The model under review builds one solid part; all positions refer to its coordinate system, in mm. Round coordinates to 2 decimals unless told otherwise and drop trailing zeros. Write each loop counter-clockwise with the first axis right and the second up, starting at its lowest first coordinate (ties: lowest second). Pieces come first, ordered by that corner, then holes. Notation, with made-up numbers: (52, 51) -> (65, 51) arc R15 ccw to (65, 76) -> close; hole circle Ø10 at (26, -19.5). An arc over 180 degrees is marked (long way). Answer in a Markdown table with one row per item. Add a question column.
```python
from build123d import *

# Parameters (mm, degrees)
SKETCH_1_W          = 213
SKETCH_1_H          = 200
EXTRUDE_1_DEPTH     = 5
SKETCH_2_R          = 2
SKETCH_2_R_2        = 6
CUT_EXTRUDE_1_DEPTH = 147.175408328
SKETCH_3_W          = 213
SKETCH_3_H          = 12.904797871
CUT_EXTRUDE_2_DEPTH = 147.175408328
SKETCH_4_W          = 28
SKETCH_4_H          = 35
CUT_EXTRUDE_3_DEPTH = 147.175408328
FILLET_1_R          = 5
SKETCH_5_W          = 42
SKETCH_5_H          = 70.904797871
EXTRUDE_2_DEPTH     = 5
FILLET_2_R          = 20
SKETCH_6_R          = 2
CUT_EXTRUDE_4_DEPTH = 202.434108173
SKETCH_7_R          = 2
CUT_EXTRUDE_5_DEPTH = 202.434108173
SKETCH_8_W          = 20
SKETCH_8_H          = 22
CUT_EXTRUDE_6_DEPTH = 202.434108173
FILLET_3_R          = 3
SKETCH_9_W          = 18
SKETCH_9_H          = 22
CUT_EXTRUDE_7_DEPTH = 202.434108173
SKETCH_10_R         = 1.5
CUT_EXTRUDE_8_DEPTH = 202.434108173
FILLET_4_R          = 10
SKETCH_11_W         = 115
SKETCH_11_H         = 73
CUT_EXTRUDE_9_DEPTH = 202.434108173
FILLET_5_R          = 5


with BuildPart() as part:
    # 草图1 → 凸台-拉伸1 (new body)
    with BuildSketch(Plane(origin=(0, 0, 0), x_dir=(1, 0, 0), z_dir=(0, 1, 0))):
        Rectangle(SKETCH_1_W, SKETCH_1_H)
    extrude(amount=EXTRUDE_1_DEPTH)

    # 草图2 → 切除-拉伸1 (cut, through all)
    with BuildSketch(Plane(origin=(0, 5, 0), x_dir=(1, 0, 0), z_dir=(0, 1, 0))):
        with Locations(Location((-4.5, 93, 0), (0, 0, 270))):
            Circle(SKETCH_2_R)
        with Locations(Location((51.5, 93, 0), (0, 0, 270))):
            Circle(SKETCH_2_R)
        with Locations(Location((-4.5, 63, 0), (0, 0, 270))):
            Circle(SKETCH_2_R)
        with Locations(Location((51.5, 63, 0), (0, 0, 270))):
            Circle(SKETCH_2_R)
        with Locations(Location((-26.5, -33.095202129, 0), (0, 0, 270))):
            Circle(SKETCH_2_R)
        with Locations(Location((29.5, -33.095202129, 0), (0, 0, 270))):
            Circle(SKETCH_2_R)
        with Locations(Location((29.5, -63.095202129, 0), (0, 0, 270))):
            Circle(SKETCH_2_R)
        with Locations(Location((-26.5, -63.095202129, 0), (0, 0, 270))):
            Circle(SKETCH_2_R)
        with Locations(Location((1.5, -48.095202129, 0), (0, 0, 270))):
            Circle(SKETCH_2_R_2)
        with Locations(Location((23.5, 78, 0), (0, 0, 270))):
            Circle(SKETCH_2_R_2)
    extrude(amount=-CUT_EXTRUDE_1_DEPTH, mode=Mode.SUBTRACT)

    # 草图3 → 切除-拉伸2 (cut, through all)
    with BuildSketch(Plane(origin=(0, 5, 0), x_dir=(1, 0, 0), z_dir=(0, 1, 0))):
        with Locations((0, -93.547601065)):
            Rectangle(SKETCH_3_W, SKETCH_3_H)
    extrude(amount=-CUT_EXTRUDE_2_DEPTH, mode=Mode.SUBTRACT)

    # 草图4 → 切除-拉伸3 (cut, through all)
    with BuildSketch(Plane(origin=(0, 5, 0), x_dir=(1, 0, 0), z_dir=(0, 1, 0))):
        with Locations((-92.5, 4.404797871)):
            Rectangle(SKETCH_4_W, SKETCH_4_H)
    extrude(amount=-CUT_EXTRUDE_3_DEPTH, mode=Mode.SUBTRACT)

    # 圆角1
    fillet_1_edges = [part.edges().sort_by_distance(p)[0] for p in [
        (-106.5, 2.5, 13.095202129),
        (-106.5, 2.5, -21.904797871),
        (-78.5, 2.5, -21.904797871),
        (-78.5, 2.5, 13.095202129),
    ]]
    fillet(fillet_1_edges, radius=FILLET_1_R)

    # 草图5 → 凸台-拉伸2 (add)
    with BuildSketch(Plane(origin=(0, 5, 0), x_dir=(1, 0, 0), z_dir=(0, 1, 0))):
        with Locations((-85.5, 135.452398936)):
            Rectangle(SKETCH_5_W, SKETCH_5_H)
    extrude(amount=-EXTRUDE_2_DEPTH)

    # 圆角2
    fillet_2_edges = [part.edges().sort_by_distance(p)[0] for p in [
        (-64.5, 2.5, -100),
    ]]
    fillet(fillet_2_edges, radius=FILLET_2_R)

    # 草图6 → 切除-拉伸4 (cut, through all)
    with BuildSketch(Plane(origin=(0, 5, 0), x_dir=(1, 0, 0), z_dir=(0, 1, 0))):
        with Locations(Location((-96.5, 158.904797871, 0), (0, 0, 270))):
            Circle(SKETCH_6_R)
        with Locations(Location((-71.5, 158.904797871, 0), (0, 0, 270))):
            Circle(SKETCH_6_R)
        with Locations(Location((-71.5, 63.904797871, 0), (0, 0, 270))):
            Circle(SKETCH_6_R)
        with Locations(Location((-96.5, 63.904797871, 0), (0, 0, 270))):
            Circle(SKETCH_6_R)
    extrude(amount=-CUT_EXTRUDE_4_DEPTH, mode=Mode.SUBTRACT)

    # 草图7 → 切除-拉伸5 (cut, through all)
    with BuildSketch(Plane(origin=(0, 5, 0), x_dir=(1, 0, 0), z_dir=(0, 1, 0))):
        with Locations(Location((-96.5, 111.404797871, 0), (0, 0, 270))):
            Circle(SKETCH_7_R)
        with Locations(Location((-96.5, -22.095202129, 0), (0, 0, 270))):
            Circle(SKETCH_7_R)
        with Locations(Location((-96.5, -77.095202129, 0), (0, 0, 270))):
            Circle(SKETCH_7_R)
        with Locations(Location((96.5, -52.095202129, 0), (0, 0, 270))):
            Circle(SKETCH_7_R)
        with Locations(Location((96.5, 4.404797871, 0), (0, 0, 270))):
            Circle(SKETCH_7_R)
        with Locations(Location((96.5, 89.404797871, 0), (0, 0, 270))):
            Circle(SKETCH_7_R)
        with Locations(Location((81.5, 89.404797871, 0), (0, 0, 270))):
            Circle(SKETCH_7_R)
        with Locations(Location((81.5, 4.404797871, 0), (0, 0, 270))):
            Circle(SKETCH_7_R)
        with Locations(Location((81.5, -52.095202129, 0), (0, 0, 270))):
            Circle(SKETCH_7_R)
    extrude(amount=-CUT_EXTRUDE_5_DEPTH, mode=Mode.SUBTRACT)

    # 草图8 → 切除-拉伸6 (cut, through all)
    with BuildSketch(Plane(origin=(0, 5, 0), x_dir=(1, 0, 0), z_dir=(0, 1, 0))):
        with Locations((81.5, -76.095202129)):
            Rectangle(SKETCH_8_W, SKETCH_8_H)
    extrude(amount=-CUT_EXTRUDE_6_DEPTH, mode=Mode.SUBTRACT)

    # 圆角3
    fillet_3_edges = [part.edges().sort_by_distance(p)[0] for p in [
        (91.5, 2.5, 87.095202129),
        (71.5, 2.5, 87.095202129),
        (71.5, 2.5, 65.095202129),
        (91.5, 2.5, 65.095202129),
    ]]
    fillet(fillet_3_edges, radius=FILLET_3_R)

    # 草图9 → 切除-拉伸7 (cut, through all)
    with BuildSketch(Plane(origin=(0, 5, 0), x_dir=(1, 0, 0), z_dir=(0, 1, 0))):
        with Locations((97.5, -76.095202129)):
            Rectangle(SKETCH_9_W, SKETCH_9_H)
    extrude(amount=-CUT_EXTRUDE_7_DEPTH, mode=Mode.SUBTRACT)

    # 草图10 → 切除-拉伸8 (cut, through all)
    with BuildSketch(Plane(origin=(0, 5, 0), x_dir=(1, 0, 0), z_dir=(0, 1, 0))):
        with Locations(Location((-74.5, 34.904797871, 0), (0, 0, 270))):
            Circle(SKETCH_10_R)
        with Locations(Location((-74.5, -14.095202129, 0), (0, 0, 270))):
            Circle(SKETCH_10_R)
    extrude(amount=-CUT_EXTRUDE_8_DEPTH, mode=Mode.SUBTRACT)

    # 圆角4
    fillet_4_edges = [part.edges().sort_by_distance(p)[0] for p in [
        (-106.5, 2.5, -170.904797871),
        (-64.5, 2.5, -170.904797871),
        (106.5, 2.5, 65.095202129),
        (-106.5, 2.5, 87.095202129),
        (106.5, 2.5, -100),
    ]]
    fillet(fillet_4_edges, radius=FILLET_4_R)

    # 草图11 → 切除-拉伸9 (cut, through all)
    with BuildSketch(Plane(origin=(0, 5, 0), x_dir=(1, 0, 0), z_dir=(0, 1, 0))):
        with Locations((16, 11.404797871)):
            Rectangle(SKETCH_11_W, SKETCH_11_H)
    extrude(amount=-CUT_EXTRUDE_9_DEPTH, mode=Mode.SUBTRACT)

    # 圆角5
    fillet_5_edges = [part.edges().sort_by_distance(p)[0] for p in [
        (-41.5, 2.5, 25.095202129),
        (-41.5, 2.5, -47.904797871),
        (73.5, 2.5, -47.904797871),
        (73.5, 2.5, 25.095202129),
    ]]
    fillet(fillet_5_edges, radius=FILLET_5_R)


solid = part.part
```
1. Insertion check: pin 1 Ø1.5 at (x, y) = (0, 1.5) entering from -Z; pin 2 Ø1.5 at (x, y) = (86, 2) entering from +Z; pin 3 Ø1.5 at (y, z) = (3, -135) entering from +X. Each pin has a flat end and moves straight along its axis. Give the tip position at first contact, or say it passes through.
2. Add section C-C on y = 1.6. State how many separate pieces and enclosed holes the cut face has, plus the area to 3 significant figures.
3. Mouldability with a two-part tool opening along X and no side actions: class faces 1 (the cylindrical face through (-67.352, 2.465, -167.898)), 2 (the cylindrical face through (1.76, 2.54, 42.1)), 3 (the cylindrical face through (23.764, 2.535, -83.994)), 4 (the cylindrical face through (-103.493, 2.465, -168.053)) as pulls with the +X half, pulls with the -X half, needs draft (parallel to the pull), parting line crosses it, or undercut.
4. For L1, parallel to Z at x = 2, y = 3.3; L2, parallel to Z at x = -74.5, y = 1.5; L3, parallel to X at y = 1.3, z = 62.5, list the stretches that pass through material, from the lowest coordinate up.
5. Add section D-D on z = -131. Write out the cut boundary in (x, y), plus the area to 3 significant figures.
6. Add section A-A on x = 1.5. Write out the cut boundary in (y, z).
7. Add section B-B on z = -78. Write out the cut boundary in (x, y), plus the area to 4 significant figures.
Filled in:
| question | item | result |
|---|---|---|
| 1 | pin 1 | z = -100 |
| 1 | pin 2 | z = 65.1 |
| 1 | pin 3 | x = -64.5 |
| 2 | separate pieces | 1 |
| 2 | enclosed holes | 26 |
| 2 | area | 32,200 mm² |
| 3 | face 1 | pulls with the +X half |
| 3 | face 2 | undercut |
| 3 | face 3 | undercut |
| 3 | face 4 | pulls with the -X half |
| 4 | L1 | -100 to -47.9, 25.1 to 42.12, 54.07 to 87.1 |
| 4 | L2 | -170.9 to -36.4, -33.4 to 12.6, 15.6 to 87.1 |
| 4 | L3 | -106.5 to -28.41, -24.59 to 27.59, 31.41 to 103.22 |
| 5 | outline | (-106.5, 0) -> (-64.5, 0) -> (-64.5, 5) -> (-106.5, 5) -> close |
| 5 | area | 210 mm² |
| 6 | outline | (0, -100) -> (5, -100) -> (5, -47.9) -> (0, -47.9) -> close; (0, 25.1) -> (5, 25.1) -> (5, 42.1) -> (0, 42.1) -> close; (0, 54.1) -> (5, 54.1) -> (5, 87.1) -> (0, 87.1) -> close |
| 7 | outline | (-106.5, 0) -> (17.5, 0) -> (17.5, 5) -> (-106.5, 5) -> close; (29.5, 0) -> (106.5, 0) -> (106.5, 5) -> (29.5, 5) -> close |
| 7 | area | 1,005 mm² |
